```python
from build123d import *

# Parameters (mm, degrees)
SKETCH1_W               = 50
SKETCH1_H               = 50
BOSS_EXTRUDE1_DEPTH     = 6.35
SKETCH2_R               = 15
CUT_EXTRUDE1_DEPTH      = 1
CUT_EXTRUDE1_DEPTH_BACK = 7.35
SKETCH3_R               = 2
CUT_EXTRUDE2_DEPTH      = 7.35
MIRROR2_COPY_1_SKETCH_R = 2
MIRROR2_COPY_1_DEPTH    = 7.35
LPATTERN2_COUNT         = 3
LPATTERN2_PITCH         = 49.784


with BuildPart() as part:
    # Sketch1 → Boss-Extrude1 (new body)
    with BuildSketch(Plane(origin=(0, 0, 0), x_dir=(1, 0, 0), z_dir=(0, 1, 0))):
        Rectangle(SKETCH1_W, SKETCH1_H)
    extrude(amount=BOSS_EXTRUDE1_DEPTH)

    # Sketch2 → Cut-Extrude1 (cut, two sides)
    with BuildSketch(Plane(origin=(0, 6.35, 0), x_dir=(1, 0, 0), z_dir=(0, 1, 0))) as cut_extrude1_sk:
        Circle(SKETCH2_R)
    extrude(amount=CUT_EXTRUDE1_DEPTH, mode=Mode.SUBTRACT)
    extrude(cut_extrude1_sk.sketch, amount=-CUT_EXTRUDE1_DEPTH_BACK, mode=Mode.SUBTRACT)

    # Sketch3 → Cut-Extrude2 (cut, through all)
    with BuildSketch(Plane(origin=(0, 6.35, 0), x_dir=(1, 0, 0), z_dir=(0, 1, 0))):
        with Locations((-15.5, 15.5)):
            Circle(SKETCH3_R)
    cut_extrude2 = extrude(amount=-CUT_EXTRUDE2_DEPTH, mode=Mode.SUBTRACT)

    # Mirror1: Cut-Extrude2 across plane
    add(cut_extrude2.mirror(Plane(origin=(0, 0, 0), x_dir=(0, 0, 1), z_dir=(1, 0, 0))), mode=Mode.SUBTRACT)

    # Mirror2: Cut-Extrude2 across plane
    add(cut_extrude2.mirror(Plane.XY), mode=Mode.SUBTRACT)

    # Mirror2 copy 1 sketch → Mirror2 copy 1 (cut, through all)
    with BuildSketch(Plane(origin=(0, 6.35, 0), x_dir=(-1, 0, 0), z_dir=(0, 1, 0))):
        with Locations((-15.5, 15.5)):
            Circle(MIRROR2_COPY_1_SKETCH_R)
    extrude(amount=-MIRROR2_COPY_1_DEPTH, mode=Mode.SUBTRACT)


with BuildPart() as lpattern2_1:
    # LPattern2: pattern copy
    add(part.part.moved(Location(Vector(1, 0, 0) * (1 * LPATTERN2_PITCH))))


with BuildPart() as lpattern2_2:
    # LPattern2: pattern copy
    add(part.part.moved(Location(Vector(1, 0, 0) * (2 * LPATTERN2_PITCH))))


with BuildPart() as part_1:
    add(part.part)

    # Combine1: union LPattern2_1, LPattern2_2
    add(lpattern2_1.part)
    add(lpattern2_2.part)


solid = part_1.part
```
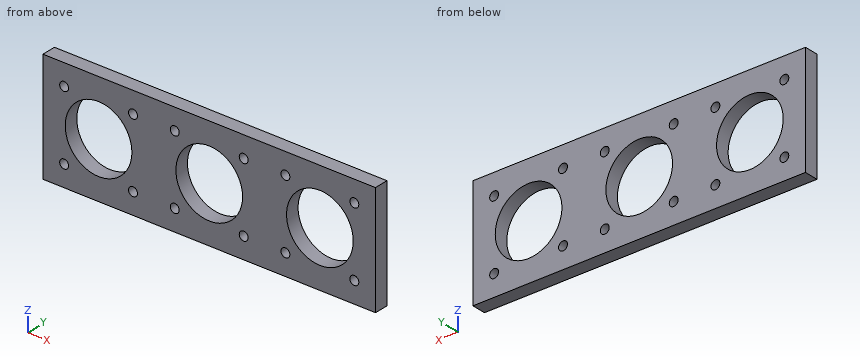
For this review, take the finished solid that the model builds, in its own axes (mm). Round coordinates to 2 decimals unless told otherwise and drop trailing zeros. Order: outer loops, then holes, each group sorted by start corner. A loop starts at its lowest first (then second) coordinate and runs counter-clockwise, first axis right, second up.
Q1. We need section C-C, the plane z = 0. Give the boundary of the cut face in (x, y), plus the area to 3 significant figures.
Findings below:
outline: (-25, 0) - (-15, 0) - (-15, 6.35) - (-25, 6.35) - close; (15, 0) - (34.78, 0) - (34.78, 6.35) - (15, 6.35) - close; (64.78, 0) - (84.57, 0) - (84.57, 6.35) - (64.78, 6.35) - close; (114.57, 0) - (124.57, 0) - (124.57, 6.35) - (114.57, 6.35) - close
area: 378 mm2
Q2. Insertion check: P1, Ø3.5, axis at x = 84.068, z = 15.5, coming from the -Y side. The pin has a flat end and moves straight along its axis. Give the tip position at first contact, or say it passes through.
Findings below:
P1: passes through
Q3. We need section A-A, the plane x = 0. Give the boundary of the cut face in (y, z).
Findings below:
outline: (0, -25) - (6.35, -25) - (6.35, -15) - (0, -15) - close; (0, 15) - (6.35, 15) - (6.35, 25) - (0, 25) - close
Q4. We need section D-D, the plane x = 99. Give the boundary of the cut face in (y, z), plus the area to 3 significant figures.
Findings below:
outline: (0, -25) - (6.35, -25) - (6.35, -14.99) - (0, -14.99) - close; (0, 14.99) - (6.35, 14.99) - (6.35, 25) - (0, 25) - close
area: 127 mm2
Q5. Wall thickness on line 1 (X direction, y = 2, z = -6.5); line 2 (Z direction, x = 15.5, y = 4.5); line 3 (X direction, y = 4.75, z = 0): over which ranges is each line inside the solid? List them lowest first.
Findings below:
line 1: x = -25 to -13.52, 13.52 to 36.27, 63.3 to 86.05, 113.09 to 124.57
line 2: z = -25 to -17.5, -13.5 to 13.5, 17.5 to 25
line 3: x = -25 to -15, 15 to 34.78, 64.78 to 84.57, 114.57 to 124.57
Q6. We need section B-B, the plane y = 1.75. State how many separate pieces and enclosed holes the cut face has, plus the area to 3 significant figures.
Findings below:
separate pieces: 1
enclosed holes: 15
area: 5,210 mm2
